Check sheet for the modelled part. Datum: model origin and axes. Units: mm. Round coordinates to 2 decimals unless told otherwise and drop trailing zeros. Order: outer loops, then holes, each group sorted by start corner. A loop starts at its lowest first (then second) coordinate and runs counter-clockwise, first axis right, second up. Notation, with made-up numbers: (8.25, 48) -> (21.25, 48) arc R19 ccw to (21.25, 57) -> close; hole circle Ø8 at (9.5, 61.5). An arc over 180 degrees is marked (long way). Use CSV: the item, a comma, the result in double quotes.
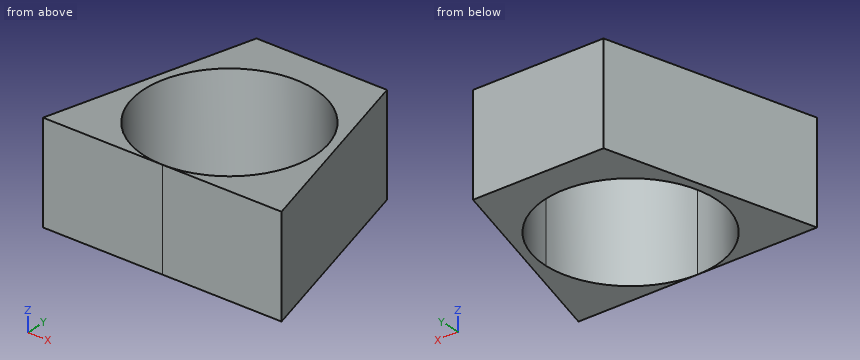
Autodesk Inventor part; units mm, degrees
ref_plane "YZ Plane" through (0, 0, 0) normal (1, 0, 0) x (0, 1, 0)
ref_plane "XZ Plane" through (0, 0, 0) normal (0, 1, 0) x (-1, 0, 0)
ref_plane "XY Plane" through (0, 0, 0) normal (0, 0, 1) x (1, 0, 0)
sketch "Sketch1" plane through (0, 0, 0) normal (0, 0, 1) x (1, 0, 0)
  circle A0 centre (0, 0) radius 8.5375
  line L0 (0, -8.5375) -> (12, -8.5375)
  line L1 (0, -8.5375) -> (-12, -8.5375)
  line L2 (-12, -8.5375) -> (-6.5648, 11.7469)
  line L3 (12, -8.5375) -> (6.5648, 11.7469)
  line L4 (12, -8.5375) -> (33, -8.5375) construction
  line L5 (6.5648, 11.7469) -> (-6.5648, 11.7469)
  dimension "d0" = 17.075
  dimension "d1" = 12
  dimension "d2" = 12
  dimension "d3" = 21
  dimension "d4" = 75
  dimension "d7" = 21
  dimension "d8" = 105
extrude "Extrusion1" add sketch "Sketch1" along normal blind 10
properties part number "parte ensamble in"
Q1. Sectioned sample at D-D, the plane y = 10.25. Enter the section's corners in (x, z).
Result sheet:
outline,"(-6.97, 0) -> (6.97, 0) -> (6.97, 10) -> (-6.97, 10) -> close"
Q2. Go/stop test with flat-tipped pins: pin 1 (4 mm diameter, centred on x = -6, y = 1.5, fed in from +Z); pin 2 (4 mm diameter, centred on y = 6.5, z = 4.5, fed in from -X); pin 3 (1 mm diameter, centred on y = -2, z = 1.5, fed in from -X). Record where each tip stops, or that it passes through.
Result sheet:
pin 1,"passes through"
pin 2,"stops at x = -8.51"
pin 3,"stops at x = -10.38"
Q3. Scan lines: L1, parallel to X at y = 0, z = 6.5; L2, parallel to X at y = 6.75, z = 5.75; L3, parallel to Y at x = -4.25, z = 8. Record each from-to range of solid material in increasing order.
Result sheet:
L1,"x = -9.71 to -8.54, 8.54 to 9.71"
L2,"x = -7.9 to -5.23, 5.23 to 7.9"
L3,"y = -8.54 to -7.4, 7.4 to 11.75"
Q4. Sectioned sample at A-A, the plane x = -7.25. Enter the section's corners in (y, z).
Result sheet:
outline,"(-8.54, 0) -> (-4.51, 0) -> (-4.51, 10) -> (-8.54, 10) -> close; (4.51, 0) -> (9.19, 0) -> (9.19, 10) -> (4.51, 10) -> close"
Q5. Sectioned sample at C-C, the plane y = -6. Enter the section's corners in (x, z).
Result sheet:
outline,"(-11.32, 0) -> (-6.07, 0) -> (-6.07, 10) -> (-11.32, 10) -> close; (6.07, 0) -> (11.32, 0) -> (11.32, 10) -> (6.07, 10) -> close"
